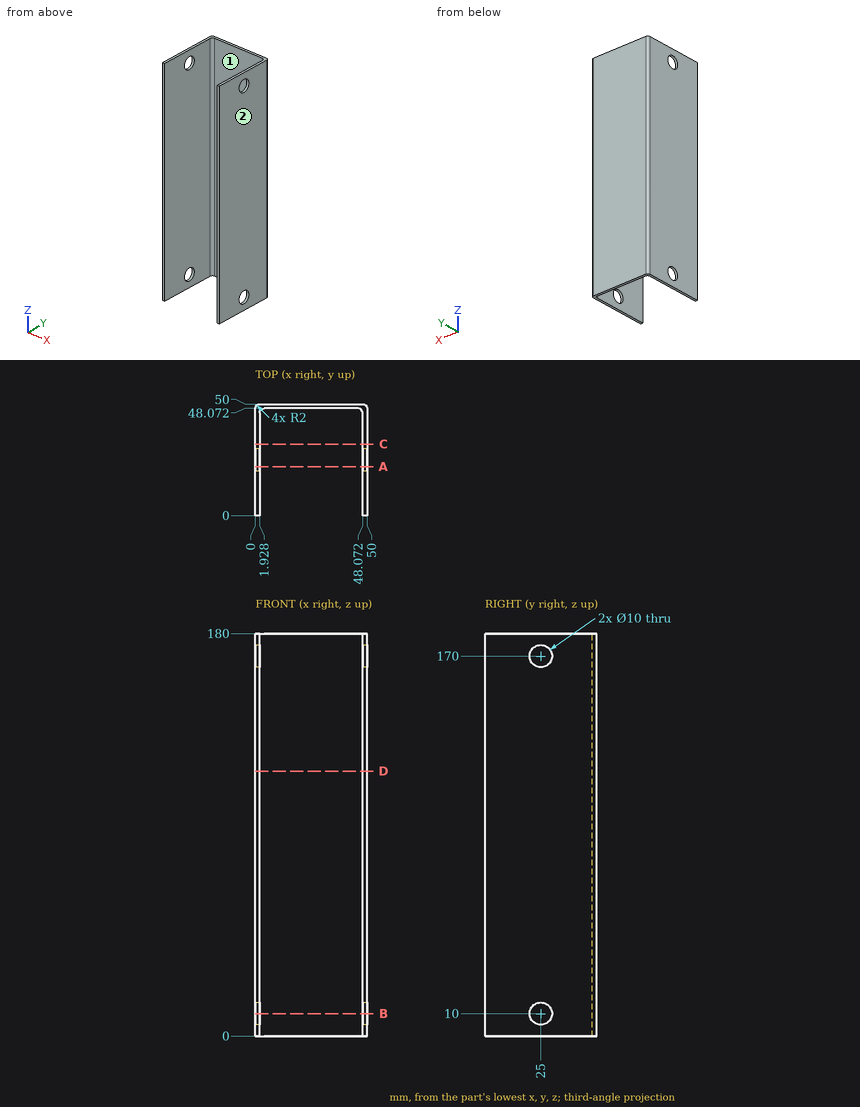
Answer from the drawing. Dimensions are ordinates in mm from the lowest x, y and z of the part. A direction names the side the tool comes from. Give positions to 0.01 mm unless a question says otherwise; leave off trailing zeros. Order: outer loops, then holes, each group sorted by start corner. A loop starts at its lowest first (then second) coordinate and runs counter-clockwise, first axis right, second up. Notation, with made-up numbers: (70.25, 68) - (123.25, 68) arc R17 ccw to (123.25, 96) - close; hole circle Ø2 at (86.5, 78). An arc over 180 degrees is marked (long way). Use one line per item in the form item = value.
1) Find section C-C on y = 32. Determine the outline of the cut face in (x, z).
Verdict:
outline = (0, 0) - (1.93, 0) - (1.93, 180) - (0, 180) - close; (48.07, 0) - (50, 0) - (50, 180) - (48.07, 180) - close
2) Find section B-B on z = 10. Determine the outline of the cut face in (x, y), and give its area (3 significant figures).
Verdict:
outline = (0, 0) - (1.93, 0) - (1.93, 20) - (0, 20) - close; (0, 30) - (1.93, 30) - (1.93, 46.07) arc R2 cw to (3.93, 48.07) - (46.07, 48.07) arc R2 cw to (48.07, 46.07) - (48.07, 30) - (50, 30) - (50, 48) arc R2 ccw to (48, 50) - (2, 50) arc R2 ccw to (0, 48) - close; (48.07, 0) - (50, 0) - (50, 20) - (48.07, 20) - close
area = 243 mm^2
3) Consider probe 1 along X at (y, z) = (4, 42.5); probe 2 along Y at (x, z) = (46.5, 150.5); probe 3 along Y at (x, z) = (14, 133.5). Determine where each line is inside the solid, lowest interval first. Write a range as [from, to].
Verdict:
probe_1 = [0, 1.93], [48.07, 50]
probe_2 = [48.03, 50]
probe_3 = [48.07, 50]
4) Find section D-D on z = 118.5. Determine the outline of the cut face in (x, y).
Verdict:
outline = (0, 0) - (1.93, 0) - (1.93, 46.07) arc R2 cw to (3.93, 48.07) - (46.07, 48.07) arc R2 cw to (48.07, 46.07) - (48.07, 0) - (50, 0) - (50, 48) arc R2 ccw to (48, 50) - (2, 50) arc R2 ccw to (0, 48) - close
5) For the marked faces 1 and 2, determine the directions among +Z, -Z, +X, -X, +Y, -Y from which every point of the face is accessible in a straight line to the end or side of a thin tool.
Verdict:
face_1 = +Z, -Z, -Y
face_2 = +Z, -Z, +X, +Y, -Y
6) Find section A-A on y = 22. Determine the outline of the cut face in (x, z).
Verdict:
outline = (0, 0) - (1.93, 0) - (1.93, 6) - (0, 6) - close; (0, 14) - (1.93, 14) - (1.93, 166) - (0, 166) - close; (0, 174) - (1.93, 174) - (1.93, 180) - (0, 180) - close; (48.07, 0) - (50, 0) - (50, 6) - (48.07, 6) - close; (48.07, 14) - (50, 14) - (50, 166) - (48.07, 166) - close; (48.07, 174) - (50, 174) - (50, 180) - (48.07, 180) - close
7) Each of these flat-tipped pins is pushed along its axis until it touches: pin 1 (6 mm diameter, centred on y = 25, z = 10, fed in from -X); pin 2 (21 mm diameter, centred on x = 33, z = 134.5, fed in from -Y). Where does it stop, or does it pass through?
Verdict:
pin_1 = through
pin_2 = 48.07
